Source: CAD feature listing. Evaluate the final solid. Frame: model axes, mm. Face numbers are marked on the shaded views. A direction names the side the tool comes from. Give positions to 0.01 mm unless a question says otherwise; leave off trailing zeros. Loops run counter-clockwise (first coordinate to the right, second up) from the corner with the lowest first, then second, coordinate; pieces in that order, holes last. Notation, with made-up numbers: (87.5, 83) -> (139.5, 83) arc R6 ccw to (139.5, 91) -> close; hole circle Ø2 at (-25.5, 17). An arc over 180 degrees is marked (long way). Answer as a JSON object with one key per item and string values. Group by question number.
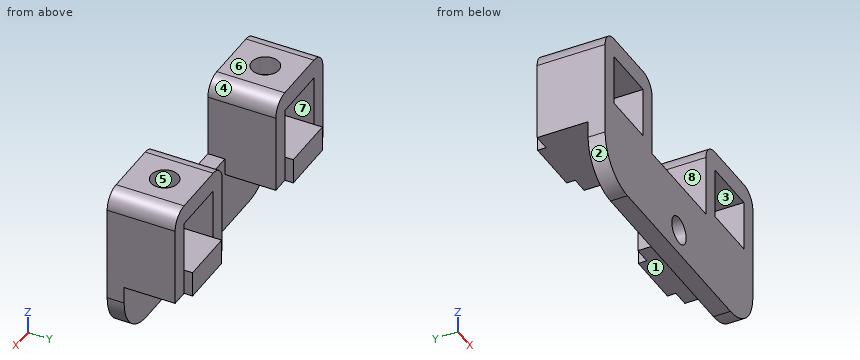
from build123d import *

# Parameters (mm, degrees)
CYLINDER077_R     = 1.6
CYLINDER077_DEPTH = 2.3
BOX189_W          = 10.5
BOX189_H          = 8
BOX189_DEPTH      = 2.3
FILLET046_R       = 2
CYLINDER078_R     = 1.6
CYLINDER078_DEPTH = 2.3
BOX190_W          = 10.5
BOX190_H          = 8
BOX190_DEPTH      = 2.3
FILLET045_R       = 2
BOX200_W          = 6.5
BOX200_H          = 9
BOX200_DEPTH      = 3
BOX199_W          = 2
BOX199_H          = 8
BOX199_DEPTH      = 9
BOX198_W          = 2
BOX198_H          = 8
BOX198_DEPTH      = 9
BOX197_W          = 6.5
BOX197_H          = 9
BOX197_DEPTH      = 3
BOX196_W          = 2
BOX196_H          = 8
BOX196_DEPTH      = 9
BOX195_W          = 2
BOX195_H          = 8
BOX195_DEPTH      = 9
CYLINDER076_R     = 1.6
CYLINDER076_DEPTH = 2
BOX194_W          = 33
BOX194_H          = 2
BOX194_DEPTH      = 9
FILLET047_R       = 5


with BuildPart() as cylinder158:
    # Cylinder077 → Cylinder077 (new body)
    with BuildSketch(Plane(origin=(47.75, 15, 6), x_dir=(1, 0, 0), z_dir=(0, 0, 1))):
        Circle(CYLINDER077_R)
    extrude(amount=CYLINDER077_DEPTH)


with BuildPart() as fillet046:
    # Box189 → Box189 (new body)
    with BuildSketch(Plane(origin=(42.5, 11, 6), x_dir=(1, 0, 0), z_dir=(0, 0, 1))):
        with Locations((5.25, 4)):
            Rectangle(BOX189_W, BOX189_H)
    extrude(amount=BOX189_DEPTH)

    # Cut100: cut Cylinder158
    add(cylinder158.part, mode=Mode.SUBTRACT)

    # Fillet046
    fillet046_edges = [fillet046.edges().sort_by_distance(p)[0] for p in [
        (42.5, 15, 8.3),
        (53, 15, 8.3),
    ]]
    fillet(fillet046_edges, radius=FILLET046_R)


with BuildPart() as cylinder159:
    # Cylinder078 → Cylinder078 (new body)
    with BuildSketch(Plane(origin=(70.25, 15, 6), x_dir=(1, 0, 0), z_dir=(0, 0, 1))):
        Circle(CYLINDER078_R)
    extrude(amount=CYLINDER078_DEPTH)


with BuildPart() as fillet045:
    # Box190 → Box190 (new body)
    with BuildSketch(Plane(origin=(65, 11, 6), x_dir=(1, 0, 0), z_dir=(0, 0, 1))):
        with Locations((5.25, 4)):
            Rectangle(BOX190_W, BOX190_H)
    extrude(amount=BOX190_DEPTH)

    # Cut101: cut Cylinder159
    add(cylinder159.part, mode=Mode.SUBTRACT)

    # Fillet045
    fillet045_edges = [fillet045.edges().sort_by_distance(p)[0] for p in [
        (65, 15, 8.3),
        (75.5, 15, 8.3),
    ]]
    fillet(fillet045_edges, radius=FILLET045_R)


with BuildPart() as cube189:
    # Box200 → Box200 (new body)
    with BuildSketch(Plane(origin=(44.5, 11, -3), x_dir=(1, 0, 0), z_dir=(0, 0, 1))):
        with Locations((3.25, 4.5)):
            Rectangle(BOX200_W, BOX200_H)
    extrude(amount=BOX200_DEPTH)


with BuildPart() as cube188:
    # Box199 → Box199 (new body)
    with BuildSketch(Plane(origin=(51, 11, -3), x_dir=(1, 0, 0), z_dir=(0, 0, 1))):
        with Locations((1, 4)):
            Rectangle(BOX199_W, BOX199_H)
    extrude(amount=BOX199_DEPTH)


with BuildPart() as cube187:
    # Box198 → Box198 (new body)
    with BuildSketch(Plane(origin=(42.5, 11, -3), x_dir=(1, 0, 0), z_dir=(0, 0, 1))):
        with Locations((1, 4)):
            Rectangle(BOX198_W, BOX198_H)
    extrude(amount=BOX198_DEPTH)


with BuildPart() as cube186:
    # Box197 → Box197 (new body)
    with BuildSketch(Plane(origin=(67, 11, -3), x_dir=(1, 0, 0), z_dir=(0, 0, 1))):
        with Locations((3.25, 4.5)):
            Rectangle(BOX197_W, BOX197_H)
    extrude(amount=BOX197_DEPTH)


with BuildPart() as cube185:
    # Box196 → Box196 (new body)
    with BuildSketch(Plane(origin=(73.5, 11, -3), x_dir=(1, 0, 0), z_dir=(0, 0, 1))):
        with Locations((1, 4)):
            Rectangle(BOX196_W, BOX196_H)
    extrude(amount=BOX196_DEPTH)


with BuildPart() as cube184:
    # Box195 → Box195 (new body)
    with BuildSketch(Plane(origin=(65, 11, -3), x_dir=(1, 0, 0), z_dir=(0, 0, 1))):
        with Locations((1, 4)):
            Rectangle(BOX195_W, BOX195_H)
    extrude(amount=BOX195_DEPTH)


with BuildPart() as cylinder157:
    # Cylinder076 → Cylinder076 (new body)
    with BuildSketch(Plane(origin=(59, 13, -7), x_dir=(1, 0, 0), z_dir=(0, -1, 0))):
        Circle(CYLINDER076_R)
    extrude(amount=CYLINDER076_DEPTH)


with BuildPart() as fusion061:
    # Box194 → Box194 (new body)
    with BuildSketch(Plane(origin=(42.5, 11, -10), x_dir=(1, 0, 0), z_dir=(0, 0, 1))):
        with Locations((16.5, 1)):
            Rectangle(BOX194_W, BOX194_H)
    extrude(amount=BOX194_DEPTH)

    # Cut102: cut Cylinder157
    add(cylinder157.part, mode=Mode.SUBTRACT)

    # Fillet047
    fillet047_edges = [fusion061.edges().sort_by_distance(p)[0] for p in [
        (42.5, 12, -10),
        (75.5, 12, -10),
    ]]
    fillet(fillet047_edges, radius=FILLET047_R)

    # Fusion061: union Fillet046, Fillet045, Cube189, Cube188, Cube187, Cube186, Cube185, Cube184
    add(fillet046.part)
    add(fillet045.part)
    add(cube189.part)
    add(cube188.part)
    add(cube187.part)
    add(cube186.part)
    add(cube185.part)
    add(cube184.part)


solid = fusion061.part
(1) First-contact query: pin 1 (0.5 mm diameter, centred on y = 19.5, z = -1, fed in from -X); pin 2 (1.5 mm diameter, centred on x = 68.5, z = -6, fed in from +Y); pin 3 (3 mm diameter, centred on x = 70, y = 16, fed in from +Z); pin 4 (4 mm diameter, centred on y = 12, z = -8, fed in from -X). Flat tips, straight axial feed; report the tip coordinate or a pass-through.
(2) Access query for the marked faces 1, 2, 3, 4 and 5. Directions: +Z, -Z, +X, -X, +Y, -Y. A direction counts if a zero-diameter tool reaches every point of the face in a straight line with its end or side. Return the directions, or none.
(3) Section query D-D on y = 15. Return the cut outline in (x, z), plus the area to 3 significant figures.
(4) Section query A-A on y = 18. Return the cut outline in (x, z), plus the area to 3 significant figures.
(5) Section query C-C on x = 45.5. Return the cut outline in (y, z).
(6) Section query B-B on z = 3.5. Return the cut outline in (x, y).
(7) Material intervals for line 1 (X direction, y = 18.25, z = 2.75); line 2 (Z direction, x = 73, y = 13.5); line 3 (Y direction, x = 47.75, z = 6.6), sorted ascending. Write a range as from..to.
(8) Mould query, pull axis Z, two halves, no side actions, for the marked faces 6, 7 and 8. Classes: pulls with the +Z half, pulls with the -Z half, needs draft (parallel to the pull), parting line crosses it, or undercut.
Result:
{
 "1": {"pin 1": "x = 44.5", "pin 2": "y = 13", "pin 3": "z = 8.3", "pin 4": "x = 42.6"},
 "2": {"face 1": "-Z, +X, -X, +Y", "face 2": "-Z, -X, +Y, -Y", "face 3": "+Y, -Y", "face 4": "+Z, +Y, -Y", "face 5": "+Z"},
 "3": {"outline": "(42.5, -3) -> (53, -3) -> (53, 6.3) arc R2 ccw to (51, 8.3) -> (49.35, 8.3) -> (49.35, 6) -> (51, 6) -> (51, 0) -> (44.5, 0) -> (44.5, 6) -> (46.15, 6) -> (46.15, 8.3) -> (44.5, 8.3) arc R2 ccw to (42.5, 6.3) -> close; (65, -3) -> (75.5, -3) -> (75.5, 6.3) arc R2 ccw to (73.5, 8.3) -> (71.85, 8.3) -> (71.85, 6) -> (73.5, 6) -> (73.5, 0) -> (67, 0) -> (67, 6) -> (68.65, 6) -> (68.65, 8.3) -> (67, 8.3) arc R2 ccw to (65, 6.3) -> close", "area": "141 mm²"},
 "4": {"outline": "(42.5, -3) -> (53, -3) -> (53, 6.3) arc R2 ccw to (51, 8.3) -> (44.5, 8.3) arc R2 ccw to (42.5, 6.3) -> close; (65, -3) -> (75.5, -3) -> (75.5, 6.3) arc R2 ccw to (73.5, 8.3) -> (67, 8.3) arc R2 ccw to (65, 6.3) -> close; hole (44.5, 0) -> (51, 0) -> (51, 6) -> (44.5, 6) -> close; hole (67, 0) -> (73.5, 0) -> (73.5, 6) -> (67, 6) -> close", "area": "156 mm²"},
 "5": {"outline": "(11, -9.58) -> (13, -9.58) -> (13, -3) -> (20, -3) -> (20, 0) -> (11, 0) -> close; (11, 6) -> (19, 6) -> (19, 8.3) -> (11, 8.3) -> close"},
 "6": {"outline": "(42.5, 11) -> (44.5, 11) -> (44.5, 19) -> (42.5, 19) -> close; (51, 11) -> (53, 11) -> (53, 19) -> (51, 19) -> close; (65, 11) -> (67, 11) -> (67, 19) -> (65, 19) -> close; (73.5, 11) -> (75.5, 11) -> (75.5, 19) -> (73.5, 19) -> close"},
 "7": {"line 1": "42.5..44.5, 51..53, 65..67, 73.5..75.5", "line 2": "-3..0, 6..8.3", "line 3": "11..13.4, 16.6..19"},
 "8": {"face 6": "pulls with the +Z half", "face 7": "undercut", "face 8": "needs draft"}
}
